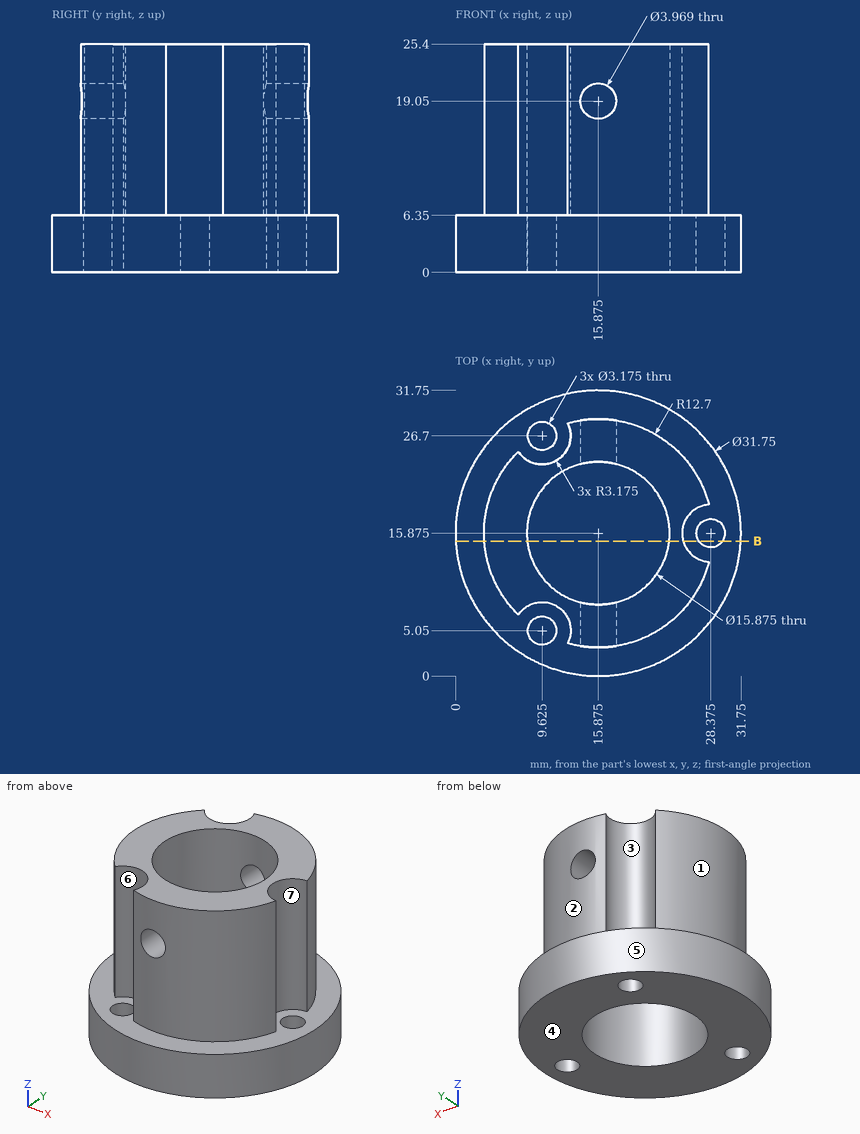
Source: three-view drawing plus pictorial views. Frame: mm from the lowest corner of the part. A direction names the side the tool comes from. Give positions to 0.01 mm unless a question says otherwise; leave off trailing zeros. Return JSON: item names as keys, results as strings.
Item 1: First-contact query: P1, Ø2, axis at x = 7.5, z = 19, coming from the +Y side; P2, Ø5, axis at x = 10, z = 4.5, coming from the +Y side; P3, Ø12, axis at y = 6.5, z = 5.5, coming from the +X side; P4, Ø5, axis at x = 17.5, y = 21.5, coming from the +Z side. Flat tips, straight axial feed; report the tip coordinate or a pass-through.
Solutions:
{"P1": "y = 24.94", "P2": "y = 31.39", "P3": "x = 31.39", "P4": "z = 25.4"}
Item 2: Access query for the marked faces 1, 2, 3 and 4. Directions: +Z, -Z, +X, -X, +Y, -Y. A direction counts if a zero-diameter tool reaches every point of the face in a straight line with its end or side. Return the directions, or none.
Solutions:
{"face 1": "+Z, -X", "face 2": "+Z, +Y", "face 3": "+Z", "face 4": "-Z, +X, -X, +Y, -Y"}
Item 3: Pull-direction query (X, two-part tool) for the marked faces 5, 6 and 7; classes: +X half, -X half, draft (parallel to the pull), parting line (faces both ways), or undercut.
Solutions:
{"face 5": "parting line", "face 6": "undercut", "face 7": "+X half"}
Item 4: Ray query, probe 1 along Y at (x, z) = (9, 1.25) (1 decimal); probe 2 along Z at (x, y) = (29.5, 23); probe 3 along Y at (x, z) = (10, 4). Return the intervals inside material, ascending.
Solutions:
{"probe 1": "1.6 to 3.6, 6.5 to 11.9, 19.8 to 25.2, 28.2 to 30.2", "probe 2": "0 to 6.35", "probe 3": "1.13 to 3.51, 6.59 to 10.54, 21.21 to 25.16, 28.24 to 30.62"}
Item 5: Cut plane B-B (y = 15). State how many separate pieces and enclosed holes the cut face has, then the cut area to 3 significant figures.
Solutions:
{"separate pieces": "3", "enclosed holes": "0", "area": "205 mm^2"}
